Can you work these out from the model? Positions are in its coordinate system, mm. Face numbers are marked on the shaded views. A direction names the side the tool comes from. Round coordinates to 2 decimals unless told otherwise and drop trailing zeros. Write each loop counter-clockwise with the first axis right and the second up, starting at its lowest first coordinate (ties: lowest second). Pieces come first, ordered by that corner, then holes.
Q1. For the marked faces 1 and 2, which set-ups out of +Z, -Z, +X, -X, +Y, -Y let a thin tool reach every point of the face, with its end or its side?
Q2. We'd pull the mould along X, two halves only. Please class the marked faces 3, 4, 5 and 6: +X half, -X half, draft (parallel to the pull), parting line (faces both ways), or undercut.
Q3. If we section it at B-B (y = 95): Please give me the cut outline in (x, z).
Q4. If we section it at A-A (z = 0): Please give me the cut outline in (x, y).
Q5. If we section it at D-D (x = -33): Please give me the cut outline in (y, z), plus the area to 3 significant figures.
Q6. If we section it at C-C (x = -24): Please give me the cut outline in (y, z).
Q7. I'm going to push flat-ended pins straight in: pin 1 Ø5 at (x, z) = (-4, 26.5) entering from +Y; pin 2 Ø3 at (y, z) = (57.5, 13.5) entering from +X; pin 3 Ø2 at (y, z) = (127, 55) entering from -X; pin 4 Ø4 at (x, z) = (24, 0) entering from +Y. Where does each tip first touch, or does it pass through?
Q8. Please list where these lines run through material, in increasing order: line 1 along X through (y, z) = (3, 0); line 2 along Z through (x, y) = (0, 72); line 3 along X through (y, z) = (131, -1).
from build123d import *

# Parameters (mm, degrees)
BOSS_EXTRUDE1_DEPTH = 150
BOSS_EXTRUDE2_DEPTH = 5
CUT_EXTRUDE2_REACH  = 172.476
SKETCH6_R           = 6.25
CUT_EXTRUDE3_REACH  = 172.476
SKETCH7_R           = 3.25


with BuildPart() as part:
    # Sketch3 → Boss-Extrude1 (new body)
    with BuildSketch(Plane(origin=(0, 0, 0), x_dir=(1, 0, 0), z_dir=(0, 1, 0))):
        with BuildLine():
            Line((-31.064919271, -71), (-38.742847032, -4.471219502))
            ThreePointArc((-38.742847032, -4.471219502), (0, 39), (38.742847032, -4.471219502))
            Line((38.742847032, -4.471219502), (31.064919271, -71))
            Line((31.064919271, -71), (0, -71))
            Line((0, -71), (-31.064919271, -71))
        make_face()
        with BuildLine():
            Line((0, -67), (-27.5, -67))
            Line((-27.5, -67), (-34.769221696, -4.012632886))
            ThreePointArc((-34.769221696, -4.012632886), (0, 35), (34.769221696, -4.012632886))
            Line((34.769221696, -4.012632886), (27.5, -67))
            Line((27.5, -67), (0, -67))
        make_face(mode=Mode.SUBTRACT)
    extrude(amount=BOSS_EXTRUDE1_DEPTH)

    # Sketch4 → Boss-Extrude2 (add)
    with BuildSketch(Plane.XZ):
        with BuildLine():
            Line((-27.5, 67), (-34.769221696, 4.012632886))
            ThreePointArc((-34.769221696, 4.012632886), (0, -35), (34.769221696, 4.012632886))
            Line((34.769221696, 4.012632886), (27.5, 67))
            Line((27.5, 67), (-27.5, 67))
        make_face()
    extrude(amount=-BOSS_EXTRUDE2_DEPTH)

    # Sketch6 → Cut-Extrude2 (cut, up to next)
    with BuildSketch(Plane.XZ, mode=Mode.PRIVATE) as cut_extrude2_sk1:
        with Locations(Location((0, 0, 0), (0, 0, 270))):
            Circle(SKETCH6_R)
    cut_extrude2_tool1 = extrude(cut_extrude2_sk1.sketch, amount=-CUT_EXTRUDE2_REACH, mode=Mode.PRIVATE) & part.part
    add(cut_extrude2_tool1.solids().sort_by_distance((0, 0, 0))[0], mode=Mode.SUBTRACT)

    # Sketch7 → Cut-Extrude3 (cut, up to next)
    with BuildSketch(Plane.XZ, mode=Mode.PRIVATE) as cut_extrude3_sk1:
        with Locations(Location((24, 0, 0), (0, 0, 270))):
            Circle(SKETCH7_R)
    cut_extrude3_tool1 = extrude(cut_extrude3_sk1.sketch, amount=-CUT_EXTRUDE3_REACH, mode=Mode.PRIVATE) & part.part
    # Sketch7 → Cut-Extrude3 (cut, up to next)
    with BuildSketch(Plane.XZ, mode=Mode.PRIVATE) as cut_extrude3_sk2:
        with Locations(Location((-24, 0, 0), (0, 0, 270))):
            Circle(SKETCH7_R)
    cut_extrude3_tool2 = extrude(cut_extrude3_sk2.sketch, amount=-CUT_EXTRUDE3_REACH, mode=Mode.PRIVATE) & part.part
    add(cut_extrude3_tool1.solids().sort_by_distance((24, 0, 0))[0], mode=Mode.SUBTRACT)
    add(cut_extrude3_tool2.solids().sort_by_distance((-24, 0, 0))[0], mode=Mode.SUBTRACT)


solid = part.part
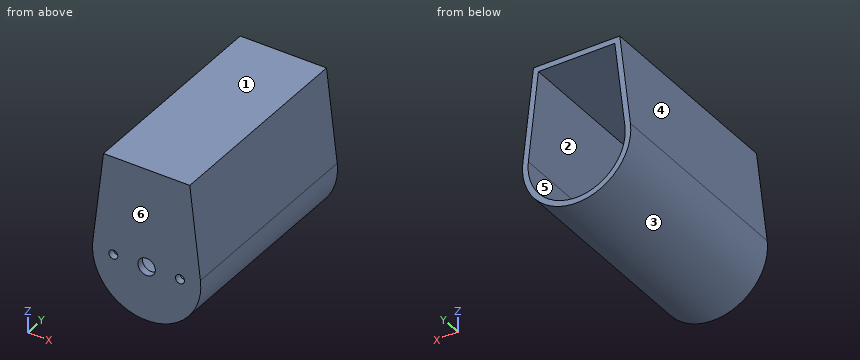
A:
1. face 1: +Z, +X, -X, +Y, -Y
1. face 2: +Y
2. face 3: parting line
2. face 4: -X half
2. face 5: undercut
2. face 6: draft
3. outline: (-38.74, 4.47) arc R39 ccw (long way) to (38.74, 4.47) - (31.06, 71) - (-31.06, 71) - close; hole (-34.77, 4.01) arc R35 ccw (long way) to (34.77, 4.01) - (27.5, 67) - (-27.5, 67) - close
4. outline: (-39, 0) - (-27.25, 0) - (-27.25, 5) - (-35, 5) - (-35, 150) - (-39, 150) - close; (-20.75, 0) - (-6.25, 0) - (-6.25, 5) - (-20.75, 5) - close; (6.25, 0) - (20.75, 0) - (20.75, 5) - (6.25, 5) - close; (27.25, 0) - (39, 0) - (39, 150) - (35, 150) - (35, 5) - (27.25, 5) - close
5. outline: (0, -20.78) - (150, -20.78) - (150, -11.66) - (5, -11.66) - (5, 19.34) - (150, 19.34) - (150, 54.23) - (0, 54.23) - close
5. area: 6,760 mm2
6. outline: (0, -30.74) - (150, -30.74) - (150, -25.48) - (5, -25.48) - (5, -3.25) - (0, -3.25) - close; (0, 3.25) - (5, 3.25) - (5, 67) - (150, 67) - (150, 71) - (0, 71) - close
7. pin 1: stops at y = 5
7. pin 2: stops at x = 37.87
7. pin 3: stops at x = -33.03
7. pin 4: passes through
8. line 1: x = -39 to -27.25, -20.75 to -6.25, 6.25 to 20.75, 27.25 to 39
8. line 2: z = -39 to -35, 67 to 71
8. line 3: x = -38.99 to -34.99, 34.99 to 38.99
